Build history of the part. All positions in model axes, mm. Face numbers are marked on the shaded views. A direction names the side the tool comes from. Coordinates: 2 decimals unless noted, no trailing zeros. Order: outer loops, then holes, each group sorted by start corner. A loop starts at its lowest first (then second) coordinate and runs counter-clockwise, first axis right, second up. Notation, with made-up numbers: (3, -5.5) - (62, -5.5) arc R34 cw to (62, 28.5) - close; hole circle Ø1 at (-29.5, -39). An arc over 180 degrees is marked (long way). Write each question's results on one line, items separated by ' | '. Start each with the question number.
from build123d import *

# Parameters (mm, degrees)
CROQUIS1_W              = 31.4
CROQUIS1_H              = 19.9
SALIENTE_EXTRUIR1_DEPTH = 5.9
CROQUIS2_R              = 1.15
SALIENTE_EXTRUIR2_DEPTH = 1.3
CROQUIS3_W              = 3.9
CROQUIS3_H              = 8.9
SALIENTE_EXTRUIR3_DEPTH = 1.3
CROQUIS4_W              = 2
CROQUIS4_H              = 0.6
SALIENTE_EXTRUIR4_DEPTH = 0.325
MATRIZL1_COUNT          = 2
MATRIZL1_PITCH          = 5.9
MATRIZL1_COUNT_DIR2     = 5
MATRIZL1_PITCH_DIR2     = 1.7
CROQUIS5_W              = 3
CROQUIS5_H              = 6.5
CORTAR_EXTRUIR1_DEPTH   = 0.325


with BuildPart() as part:
    # Croquis1 → Saliente-Extruir1 (new body)
    with BuildSketch(Plane(origin=(0, 0, 0), x_dir=(0, 0, -1), z_dir=(1, 0, 0))):
        Rectangle(CROQUIS1_W, CROQUIS1_H)
    extrude(amount=SALIENTE_EXTRUIR1_DEPTH)

    # Croquis2 → Saliente-Extruir2 (add)
    with BuildSketch(Plane.ZY):
        Polygon((21.6, 2.55), (21.6, -2.55), (20.7, -2.55), (20.7, -8.1), (-20.7, -8.1), (-20.7, -2.55), (-21.6, -2.55), (-21.6, 2.55), (-20.7, 2.55), (-20.7, 8.1), (20.7, 8.1), (20.7, 2.55), align=None)
        with Locations((-17.75, 0)):
            Circle(CROQUIS2_R, mode=Mode.SUBTRACT)
        with Locations((17.75, 0)):
            Circle(CROQUIS2_R, mode=Mode.SUBTRACT)
    extrude(amount=SALIENTE_EXTRUIR2_DEPTH)

    # Croquis3 → Saliente-Extruir3 (add)
    with BuildSketch(Plane.ZY.offset(1.3)):
        with Locations((-10.45, -0.15)):
            Rectangle(CROQUIS3_W, CROQUIS3_H)
    extrude(amount=SALIENTE_EXTRUIR3_DEPTH)

    # Croquis4 → Saliente-Extruir4 (add)
    with BuildSketch(Plane.ZY.offset(1.3)):
        with Locations((-7.5, -4.05)):
            Rectangle(CROQUIS4_W, CROQUIS4_H)
    saliente_extruir4 = extrude(amount=SALIENTE_EXTRUIR4_DEPTH)

    # MatrizL1: Saliente-Extruir4 2 × 5
    with Locations(*[(0, j * MATRIZL1_PITCH_DIR2, -i * MATRIZL1_PITCH) for i in range(MATRIZL1_COUNT) for j in range(MATRIZL1_COUNT_DIR2) if (i, j) != (0, 0)]):
        add(saliente_extruir4)

    # Croquis5 → Cortar-Extruir1 (cut)
    with BuildSketch(Plane(origin=(5.9, 0, 0), x_dir=(0, 0, -1), z_dir=(1, 0, 0))):
        Polygon((-12.7, 1.95), (-12.7, 5.45), (10.5, 5.45), (10.5, 2.45), (11.8, 2.45), (11.8, -2.45), (10.5, -2.45), (10.5, -5.45), (-12.7, -5.45), (-12.7, -1.95), (-11.4, -1.95), (-11.4, -4.15), (9.2, -4.15), (9.2, -1.15), (9.2, 1.15), (9.2, 4.15), (-11.4, 4.15), (-11.4, 1.95), align=None)
        with Locations((1.2, 0)):
            Rectangle(CROQUIS5_W, CROQUIS5_H)
        with Locations((5.8, 0)):
            Rectangle(CROQUIS5_W, CROQUIS5_H)
        with Locations((-3.4, 0)):
            Rectangle(CROQUIS5_W, CROQUIS5_H)
        with Locations((-8, 0)):
            Rectangle(CROQUIS5_W, CROQUIS5_H)
    extrude(amount=-CORTAR_EXTRUIR1_DEPTH, mode=Mode.SUBTRACT)


solid = part.part
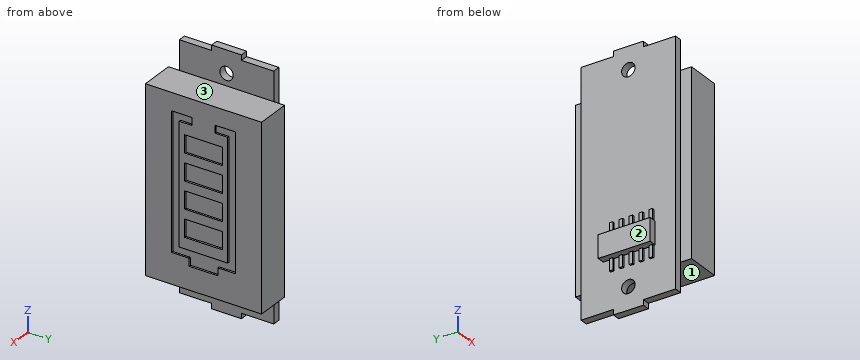
Item 1: Slice it at B-B (x = -0.5). Write the cut outline in (y, z).
Item 2: Which spindle directions (+Z, -Z, +X, -X, +Y, -Y) get a long thin tool onto all of the face, cutting with end or side? Do the marked faces 1, 2 and 3. Say none if no direction does.
Item 3: Probe probe 1 along Y at (x, z) = (-0.9, -17.75); probe 2 along X at (y, z) = (8.5, -10.5); probe 3 along X at (y, z) = (4, -10) (3 decimals). List the from-to ranges inside material, lowest first.
Item 4: Slice it at D-D (x = 2.25). Write the cut outline in (y, z).
Item 5: Flat gauge pins, fed straight in: P1, Ø3, axis at x = -1.5, y = 7, coming from the -Z side; P2, Ø1, axis at y = -1.5, z = -2.5, coming from the -X side; P3, Ø5, axis at x = 4, y = 2.5, coming from the +Z side. Where does each tip first touch, or does it go through?
Item 6: Slice it at A-A (z = 17.75). Write the cut outline in (x, y).
Item 7: Slice it at C-C (z = -14). Write the cut outline in (x, y) (3 decimals), then the cut area to 3 significant figures.
Resolved:
1) outline: (-8.1, -20.7) - (-2.55, -20.7) - (-2.55, -21.6) - (2.55, -21.6) - (2.55, -20.7) - (8.1, -20.7) - (8.1, 20.7) - (2.55, 20.7) - (2.55, 21.6) - (-2.55, 21.6) - (-2.55, 20.7) - (-8.1, 20.7) - close; hole circle Ø2.3 at (0, -17.75); hole circle Ø2.3 at (0, 17.75)
2) face 1: -Z, +X, +Y, -Y | face 2: +Z, -Z, -X, +Y, -Y | face 3: +Z, +X, +Y, -Y
3) probe 1: -8.1 to -1.15, 1.15 to 8.1 | probe 2: 0 to 5.9 | probe 3: -2.6 to 5.575
4) outline: (-9.95, -15.7) - (9.95, -15.7) - (9.95, 15.7) - (-9.95, 15.7) - close
5) P1: z = -20.7 | P2: x = -1.3 | P3: z = 15.7
6) outline: (-1.3, -8.1) - (0, -8.1) - (0, -1.15) - (-1.3, -1.15) - close; (-1.3, 1.15) - (0, 1.15) - (0, 8.1) - (-1.3, 8.1) - close
7) outline: (-1.625, -4.35) - (-1.3, -4.35) - (-1.3, -8.1) - (0, -8.1) - (0, -9.95) - (5.9, -9.95) - (5.9, 9.95) - (0, 9.95) - (0, 8.1) - (-1.3, 8.1) - (-1.3, 3.05) - (-1.625, 3.05) - (-1.625, 2.45) - (-1.3, 2.45) - (-1.3, 1.35) - (-1.625, 1.35) - (-1.625, 0.75) - (-1.3, 0.75) - (-1.3, -0.35) - (-1.625, -0.35) - (-1.625, -0.95) - (-1.3, -0.95) - (-1.3, -2.05) - (-1.625, -2.05) - (-1.625, -2.65) - (-1.3, -2.65) - (-1.3, -3.75) - (-1.625, -3.75) - close | area: 139 mm^2
